Can you work these out from the drawing? Everything is in mm from the part's minimum corner. Round coordinates to 2 decimals unless told otherwise and drop trailing zeros. Write each loop counter-clockwise with the first axis right and the second up, starting at its lowest first coordinate (ties: lowest second). Pieces come first, ordered by that corner, then holes. Notation, with made-up numbers: M 23.5,39 L 36.5,39 A15 ccw 36.5,44 Z; hole C 63,35.5 d9. An arc over 180 degrees is marked long. Answer in a Markdown table with one row per item. Add a question column.
(1) If I drill on probe 1 along X at (y, z) = (6.75, 2.15); probe 2 along Y at (x, z) = (114, 3.2); probe 3 along X at (y, z) = (1, 0.3), over which ranges is the centre line in solid material (lowest first)?
(2) Suppose I cut it at A-A, the plane x = 115. Write out the boundary of the cut face in (y, z), then the cut area to 3 significant figures.
(3) Suppose I cut it at B-B, the plane z = 3.5. Write out the boundary of the cut face in (x, y), then the cut area to 3 significant figures.
(4) Suppose I cut it at C-C, the plane y = 7.5. Write out the boundary of the cut face in (x, z).
(5) I'm going to push a flat-ended pin straight in: pin 1 (4.5 mm diameter, centred on x = 5, y = 7.5, fed in from -Z). Where does the tip first touch, or does it pass through?
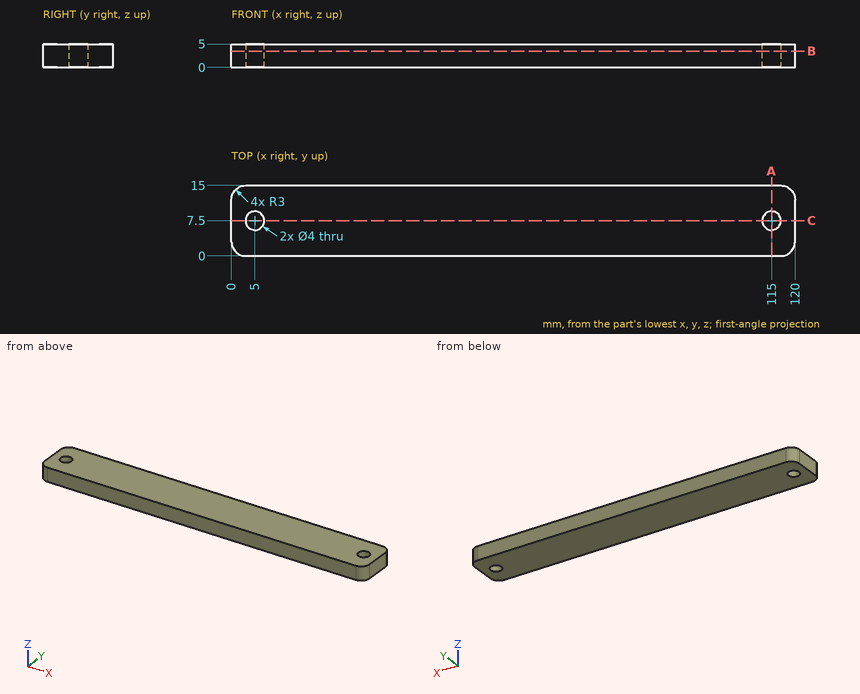
Calculated:
| question | item | result |
|---|---|---|
| 1 | probe 1 | 0 to 3.15, 6.85 to 113.15, 116.85 to 120 |
| 1 | probe 2 | 0 to 5.77, 9.23 to 15 |
| 1 | probe 3 | 0.76 to 119.24 |
| 2 | outline | M 0,0 L 5.5,0 L 5.5,5 L 0,5 Z; M 9.5,0 L 15,0 L 15,5 L 9.5,5 Z |
| 2 | area | 55.0 mm² |
| 3 | outline | M 0,3 A3 ccw 3,0 L 117,0 A3 ccw 120,3 L 120,12 A3 ccw 117,15 L 3,15 A3 ccw 0,12 Z; hole C 5,7.5 d4; hole C 115,7.5 d4 |
| 3 | area | 1,770 mm² |
| 4 | outline | M 0,0 L 3,0 L 3,5 L 0,5 Z; M 7,0 L 113,0 L 113,5 L 7,5 Z; M 117,0 L 120,0 L 120,5 L 117,5 Z |
| 5 | pin 1 | z = 0 |
